The figure shows three views and two pictorial views of one solid part (mm, origin at its lowest corner). Answer the questions. A direction names the side the tool comes from. Coordinates: 2 decimals unless noted, no trailing zeros. Write each loop counter-clockwise with the first axis right and the second up, starting at its lowest first coordinate (ties: lowest second). Pieces come first, ordered by that corner, then holes.
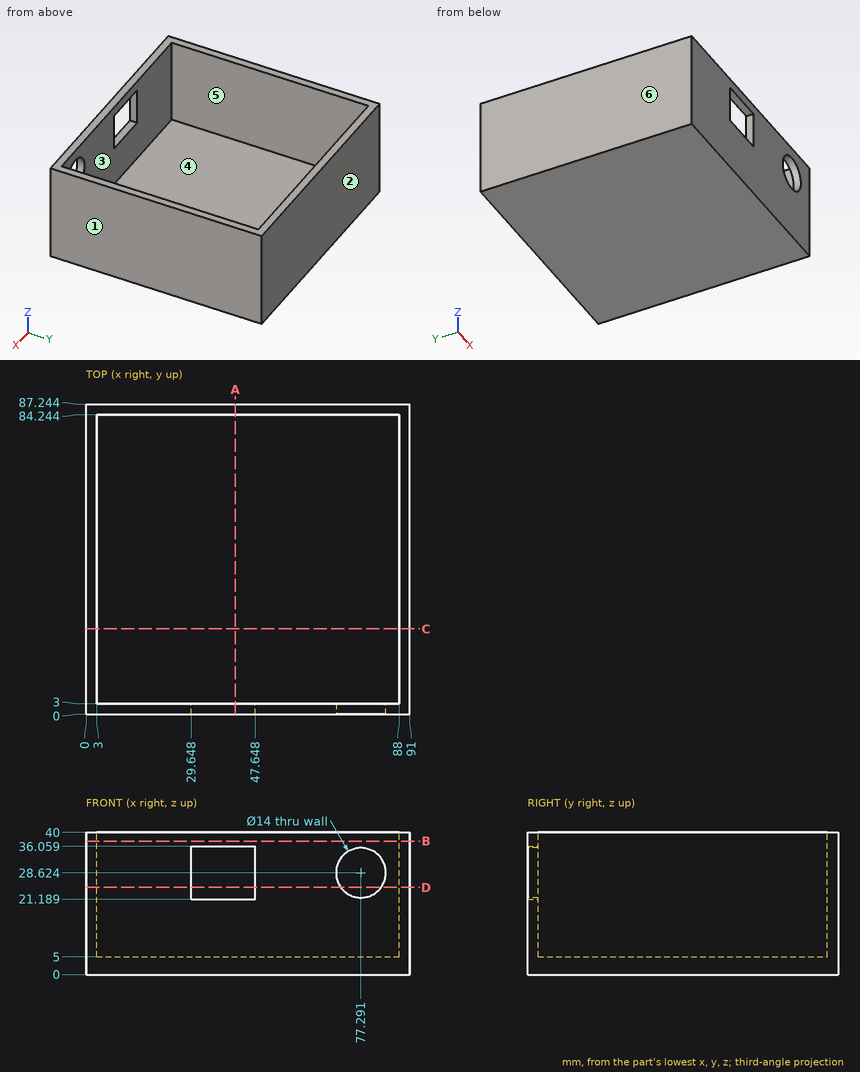
Item 1: Find the intervals of material crossed by probe 1 along X at (y, z) = (56, 7); probe 2 along Y at (x, z) = (43, 21) (1 decimal); probe 3 along Z at (x, y) = (65.5, 22), in increasing order.
Item 2: For the marked faces 5 and 6, determine the directions among +Z, -Z, +X, -X, +Y, -Y from which every point of the face is accessible in a straight line to the end or side of a thin tool.
Item 3: Given pin 1 (11 mm diameter, centred on x = 77.29, z = 28.62, fed in from -Y); pin 2 (5 mm diameter, centred on x = 31, y = 68.5, fed in from +Z), each flat-ended and moving along its own axis, determine where each tip first touches the part or whether it passes through.
Item 4: The part is cut by section D-D (z = 24.5). Give the vertices of the cut face in (x, y) (1 decimal).
Item 5: The part is cut by section C-C (y = 24). Give the vertices of the cut face in (x, z).
Item 6: The part is cut by section B-B (z = 37.5). Give the vertices of the cut face in (x, y) (1 decimal), and give its area (3 significant figures).
Item 7: The part is cut by section A-A (x = 42). Give the vertices of the cut face in (y, z) (1 decimal).
Item 8: Determine the mould class of the marked faces 1, 2, 3 and 4 for opening direction X: +X half, -X half, draft (parallel to the pull), parting line (faces both ways), or undercut.
Answer:
1. probe 1: x = 0 to 3, 88 to 91
1. probe 2: y = 0 to 3, 84.2 to 87.2
1. probe 3: z = 0 to 5
2. face 5: +Z
2. face 6: +Z, -Z, -X, +Y, -Y
3. pin 1: stops at y = 84.24
3. pin 2: stops at z = 5
4. outline: (0, 0) - (29.6, 0) - (29.6, 3) - (3, 3) - (3, 84.2) - (88, 84.2) - (88, 3) - (82.9, 3) - (82.9, 0) - (91, 0) - (91, 87.2) - (0, 87.2) - close; (47.6, 0) - (71.6, 0) - (71.6, 3) - (47.6, 3) - close
5. outline: (0, 0) - (91, 0) - (91, 40) - (88, 40) - (88, 5) - (3, 5) - (3, 40) - (0, 40) - close
6. outline: (0, 0) - (91, 0) - (91, 87.2) - (0, 87.2) - close; hole (3, 3) - (88, 3) - (88, 84.2) - (3, 84.2) - close
6. area: 1,030 mm2
7. outline: (0, 0) - (87.2, 0) - (87.2, 40) - (84.2, 40) - (84.2, 5) - (3, 5) - (3, 21.2) - (0, 21.2) - close; (0, 36.1) - (3, 36.1) - (3, 40) - (0, 40) - close
8. face 1: +X half
8. face 2: draft
8. face 3: undercut
8. face 4: undercut
